Could you check a few things on this drawing? It's one solid part, dimensions in mm from its lowest x, y, z. A direction names the side the tool comes from. Round coordinates to 2 decimals unless told otherwise and drop trailing zeros. Write each loop counter-clockwise with the first axis right and the second up, starting at its lowest first coordinate (ties: lowest second). Pieces come first, ordered by that corner, then holes. Notation, with made-up numbers: (55, -15.5) -> (76, -15.5) arc R34 cw to (76, 21.5) -> close; hole circle Ø1 at (35.5, -34). An arc over 180 degrees is marked (long way). Answer in a Markdown table with one row per item. Add a question column.
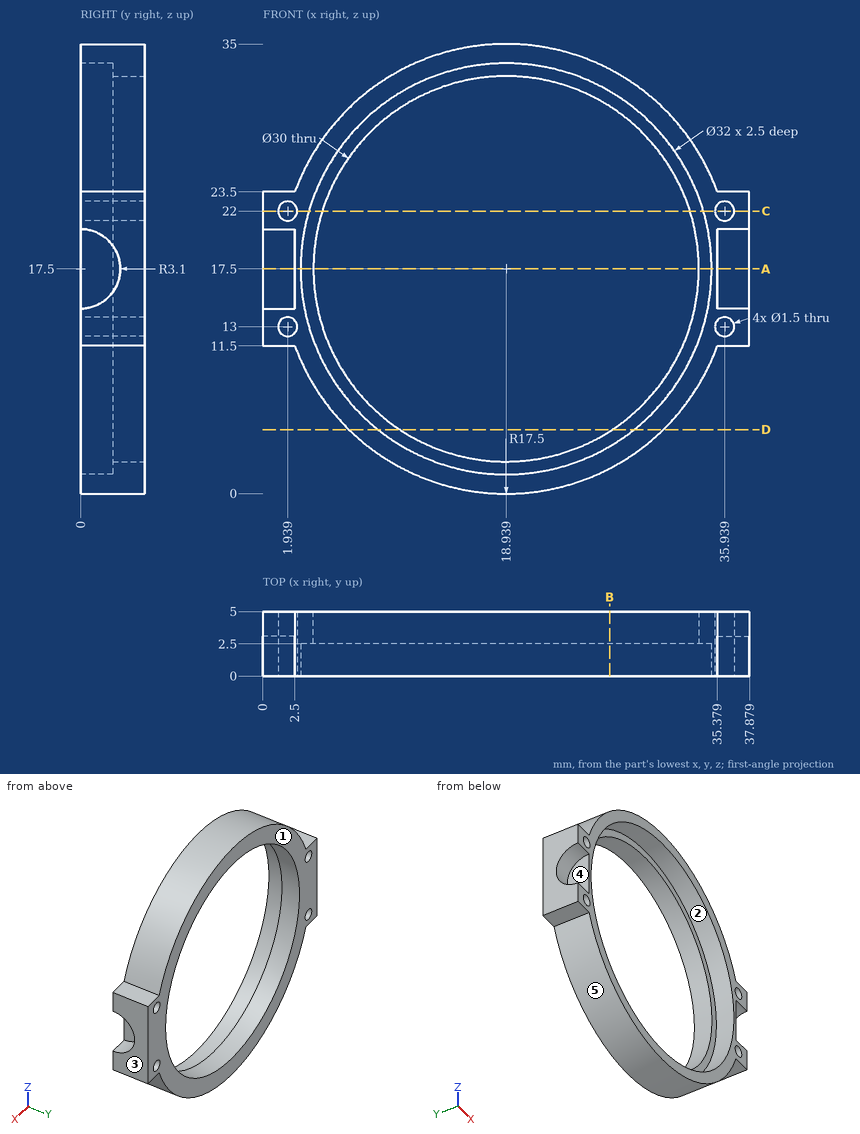
Item 1: If we section it at A-A on z = 17.5: Please give me the cut outline in (x, y), then the cut area to 3 significant figures.
Item 2: On a 3-axis mill with a long thin cutter (end or side, diameter ignored), from which of +Z, -Z, +X, -X, +Y, -Y can I reach the whole of each face in a straight line? I mean the marked faces 4 and 5. Say none if no direction works.
Item 3: If we section it at B-B on x = 27: Please give me the cut outline in (y, z).
Item 4: For P1, Ø1.2, axis at x = 37, y = 2.5, coming from the -Z side; P2, Ø1.6, axis at y = 1, z = 19, coming from the -X side; P3, Ø0.8, axis at x = 1, y = 3.5, coming from the +Z side, each with a flat end and sliding along its axis, tell me the tip position at first contact or that it passes through.
Item 5: If we section it at D-D on z = 5: Please give me the cut outline in (x, y).
Item 6: If we mould it in two halves opening along X, with no side actions, what happens to the marked faces 1, 2 and 3? For each: pulls with the +X half, pulls with the -X half, needs draft (parallel to the pull), parting line crosses it, or undercut.
Item 7: If we section it at C-C on z = 22: Please give me the cut outline in (x, y) (1 decimal).
Item 8: I need wall thicknesses on line 1 along Z through (x, y) = (2, 3.5); line 2 along Z through (x, y) = (36.5, 4.1); line 3 along X through (y, z) = (3.9, 13). Which ranges of each line are inside material? Lowest first, please. Write a range as from..to.
Results list:
| question | item | result |
|---|---|---|
| 1 | outline | (0, 3.1) -> (2.5, 3.1) -> (2.5, 0) -> (2.94, 0) -> (2.94, 2.5) -> (3.94, 2.5) -> (3.94, 5) -> (0, 5) -> close; (33.94, 2.5) -> (34.94, 2.5) -> (34.94, 0) -> (35.38, 0) -> (35.38, 3.1) -> (37.88, 3.1) -> (37.88, 5) -> (33.94, 5) -> close |
| 1 | area | 18.9 mm² |
| 2 | face 4 | -X, -Y |
| 2 | face 5 | -Z, +Y, -Y |
| 3 | outline | (0, 1.97) -> (5, 1.97) -> (5, 4.85) -> (2.5, 4.85) -> (2.5, 3.68) -> (0, 3.68) -> close; (0, 31.32) -> (2.5, 31.32) -> (2.5, 30.15) -> (5, 30.15) -> (5, 33.03) -> (0, 33.03) -> close |
| 4 | P1 | z = 11.5 |
| 4 | P2 | x = 2.5 |
| 4 | P3 | z = 23.5 |
| 5 | outline | (6.69, 0) -> (8.95, 0) -> (8.95, 2.5) -> (10.65, 2.5) -> (10.65, 5) -> (6.69, 5) -> close; (27.23, 2.5) -> (28.93, 2.5) -> (28.93, 0) -> (31.19, 0) -> (31.19, 5) -> (27.23, 5) -> close |
| 6 | face 1 | needs draft |
| 6 | face 2 | undercut |
| 6 | face 3 | pulls with the +X half |
| 7 | outline | (0, 0) -> (1.2, 0) -> (1.2, 5) -> (0, 5) -> close; (2.7, 0) -> (3.6, 0) -> (3.6, 2.5) -> (4.6, 2.5) -> (4.6, 5) -> (2.7, 5) -> close; (33.2, 2.5) -> (34.3, 2.5) -> (34.3, 0) -> (35.2, 0) -> (35.2, 5) -> (33.2, 5) -> close; (36.7, 0) -> (37.9, 0) -> (37.9, 5) -> (36.7, 5) -> close |
| 8 | line 1 | 11.5..12.25, 13.75..21.25, 22.75..23.5 |
| 8 | line 2 | 11.5..12.5, 13.5..21.5, 22.5..23.5 |
| 8 | line 3 | 0..1.19, 2.69..4.63, 33.25..35.19, 36.69..37.88 |
